```python
from build123d import *

# Parameters (mm, degrees)
BOSS_EXTRUDE1_DEPTH = 12.7
CUT_EXTRUDE1_REACH  = 45.562
SKETCH2_R           = 3.175
CUT_EXTRUDE2_REACH  = 44.17
SKETCH3_R           = 3.175


with BuildPart() as part:
    # Sketch1 → Boss-Extrude1 (new, symmetric)
    with BuildSketch(Plane.XY):
        Polygon((0, 39.6875), (0, 15.875), (6.477, 15.875), (6.477, -15.875), (0, -15.875), (0, -39.6875), (12.7, -39.6875), (12.7, 39.6875), align=None)
    extrude(amount=BOSS_EXTRUDE1_DEPTH, both=True)

    # Sketch2 → Cut-Extrude1 (cut, up to next)
    with BuildSketch(Plane.ZY, mode=Mode.PRIVATE) as cut_extrude1_sk1:
        with Locations(Location((0, 26.9875, 0), (0, 0, 270))):
            Circle(SKETCH2_R)
    cut_extrude1_tool1 = extrude(cut_extrude1_sk1.sketch, amount=-CUT_EXTRUDE1_REACH, mode=Mode.PRIVATE) & part.part
    cut_extrude1 = cut_extrude1_tool1.solids().sort_by_distance((0, 26.9875, 0))[0]
    add(cut_extrude1, mode=Mode.SUBTRACT)

    # Mirror1: Cut-Extrude1 across plane
    add(cut_extrude1.mirror(Plane.ZX), mode=Mode.SUBTRACT)

    # Sketch3 → Cut-Extrude2 (cut, up to next)
    with BuildSketch(Plane.ZY.offset(-6.477), mode=Mode.PRIVATE) as cut_extrude2_sk1:
        with Locations((0, 8.4963)):
            Circle(SKETCH3_R)
    cut_extrude2_tool1 = extrude(cut_extrude2_sk1.sketch, amount=-CUT_EXTRUDE2_REACH, mode=Mode.PRIVATE) & part.part
    # Sketch3 → Cut-Extrude2 (cut, up to next)
    with BuildSketch(Plane.ZY.offset(-6.477), mode=Mode.PRIVATE) as cut_extrude2_sk2:
        with Locations((0, -8.4963)):
            Circle(SKETCH3_R)
    cut_extrude2_tool2 = extrude(cut_extrude2_sk2.sketch, amount=-CUT_EXTRUDE2_REACH, mode=Mode.PRIVATE) & part.part
    # Sketch3 → Cut-Extrude2 (cut, up to next)
    with BuildSketch(Plane.ZY.offset(-6.477), mode=Mode.PRIVATE) as cut_extrude2_sk3:
        with Locations((6.908794346, 0.0125)):
            Circle(SKETCH3_R)
    cut_extrude2_tool3 = extrude(cut_extrude2_sk3.sketch, amount=-CUT_EXTRUDE2_REACH, mode=Mode.PRIVATE) & part.part
    # Sketch3 → Cut-Extrude2 (cut, up to next)
    with BuildSketch(Plane.ZY.offset(-6.477), mode=Mode.PRIVATE) as cut_extrude2_sk4:
        with Locations((-6.908805654, 0)):
            Circle(SKETCH3_R)
    cut_extrude2_tool4 = extrude(cut_extrude2_sk4.sketch, amount=-CUT_EXTRUDE2_REACH, mode=Mode.PRIVATE) & part.part
    add(cut_extrude2_tool1.solids().sort_by_distance((6.477, 8.4963, 0))[0], mode=Mode.SUBTRACT)
    add(cut_extrude2_tool2.solids().sort_by_distance((6.477, -8.4963, 0))[0], mode=Mode.SUBTRACT)
    add(cut_extrude2_tool3.solids().sort_by_distance((6.477, 0.0125, 6.908794))[0], mode=Mode.SUBTRACT)
    add(cut_extrude2_tool4.solids().sort_by_distance((6.477, 0, -6.908806))[0], mode=Mode.SUBTRACT)


solid = part.part
```
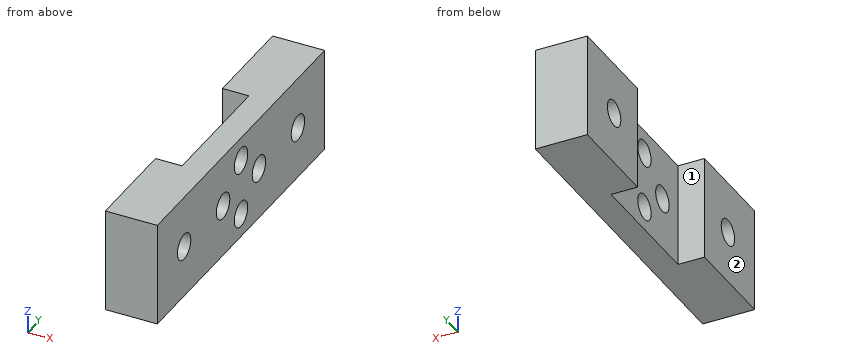
The listing builds one solid part. Answer for the finished solid, in the listing's coordinates (mm). Face numbers are marked on the shaded views. A direction names the side the tool comes from. Give positions to 0.01 mm unless a question says otherwise; leave off trailing zeros. Loops run counter-clockwise (first coordinate to the right, second up) from the corner with the lowest first, then second, coordinate; pieces in that order, holes last. Notation, with made-up numbers: M 73,78.25 L 89,78.25 A18 ccw 89,98.25 Z; hole C 88.5,4.25 d10. An arc over 180 degrees is marked long. One line per item, written item: value.
Q1. A flat-ended cylindrical pin translates along its axis: P1, Ø12.5, axis at y = -3, z = -2, coming from the -X side. Find the tip coordinate at first contact, or state that the pin passes through.
Working result:
P1: stops at x = 6.48
Q2. A cutting plane is placed at C-C on y = -25.5. Determine the outline of the cut face in (x, z), then the cut area to 3 significant figures.
Working result:
outline: M 0,-12.7 L 12.7,-12.7 L 12.7,-2.8 L 0,-2.8 Z; M 0,2.8 L 12.7,2.8 L 12.7,12.7 L 0,12.7 Z
area: 251 mm^2
Q3. A cutting plane is placed at A-A on x = 1. Give the number of separate pieces and of enclosed holes in the cut face, then the cut area to 3 significant figures.
Working result:
separate pieces: 2
enclosed holes: 2
area: 1,150 mm^2
Q4. A cutting plane is placed at D-D on z = 11. Determine the outline of the cut face in (x, y) (1 decimal), then the cut area to 3 significant figures.
Working result:
outline: M 0,-39.7 L 12.7,-39.7 L 12.7,39.7 L 0,39.7 L 0,15.9 L 6.5,15.9 L 6.5,-15.9 L 0,-15.9 Z
area: 802 mm^2
Q5. A cutting plane is placed at B-B on z = 0. Determine the outline of the cut face in (x, y) (1 decimal).
Working result:
outline: M 0,-39.7 L 12.7,-39.7 L 12.7,-30.2 L 0,-30.2 Z; M 0,-23.8 L 12.7,-23.8 L 12.7,-11.7 L 6.5,-11.7 L 6.5,-15.9 L 0,-15.9 Z; M 0,15.9 L 6.5,15.9 L 6.5,11.7 L 12.7,11.7 L 12.7,23.8 L 0,23.8 Z; M 0,30.2 L 12.7,30.2 L 12.7,39.7 L 0,39.7 Z; M 6.5,-5.3 L 12.7,-5.3 L 12.7,5.3 L 6.5,5.3 Z
Q6. For the marked faces 1 and 2, determine the directions among +Z, -Z, +X, -X, +Y, -Y from which every point of the face is accessible in a straight line to the end or side of a thin tool.
Working result:
face 1: +Z, -Z, -X
face 2: +Z, -Z, -X, +Y, -Y
Q7. Find the intervals of material crossed by line 1 (Z direction, x = 10.25, y = 27); line 2 (Y direction, x = 2.75, z = 1.25) (1 decimal); line 3 (Y direction, x = 8, z = 0.5), in increasing order. Write a range as from..to.
Working result:
line 1: z = -12.7..-3.17, 3.17..12.7
line 2: y = -39.7..-29.9, -24.1..-15.9, 15.9..24.1, 29.9..39.7
line 3: y = -39.69..-30.12, -23.85..-11.63, -5.36..5.36, 11.63..23.85, 30.12..39.69
